For this review, use the dimensioned drawing (mm, ordinates from the lowest corner) and the shaded views. A direction names the side the tool comes from. Coordinates: 2 decimals unless noted, no trailing zeros. Loops run counter-clockwise (first coordinate to the right, second up) from the corner with the lowest first, then second, coordinate; pieces in that order, holes last. Notation, with made-up numbers: (-1, -37.75) - (16, -37.75) arc R23 cw to (16, -7.75) - close; hole circle Ø5 at (-0.5, -36). An arc over 180 degrees is marked (long way). Use one line per item in the form item = value. Start each with the question number.
(1) Clearance check with flat-ended pins moving along their axes: pin 1 Ø3 at (y, z) = (5.5, 25.5) entering from +X; pin 2 Ø0.9 at (x, z) = (16, 8.5) entering from +Y; pin 3 Ø3 at (x, z) = (16.5, 15) entering from -Y. State where each tip first meets the part, or that it passes through.
(2) Add section C-C (z = 23.75). State the section outline as (x, y) points.
(3) The part is to be moulded in two halves that separate along Z. For the marked faces 4, 5 and 6, say which applies: pulls with the +Z half, pulls with the -Z half, needs draft (parallel to the pull), parting line crosses it, or undercut.
(4) Add section D-D (y = 6.75). State the section outline as (x, z) points, plus the area to 3 significant figures.
(5) Tool access review of the marked faces 1, 2 and 3: name each direction out of +Z, -Z, +X, -X, +Y, -Y from which nothing blocks a thin tool from reaching the whole face with its end or side.
(6) Add section B-B (x = 16.5). State the section outline as (y, z) points, plus the area to 3 significant figures.
(7) For L1, parallel to Z at x = 16.5, y = 4.5; L2, parallel to Z at x = 16.5, y = 6.6; L3, parallel to X at y = 4, z = 15, list the stretches that pass through material, from the lowest coordinate up.
(8) Add section A-A (y = 4.5). State the section outline as (x, z) points.
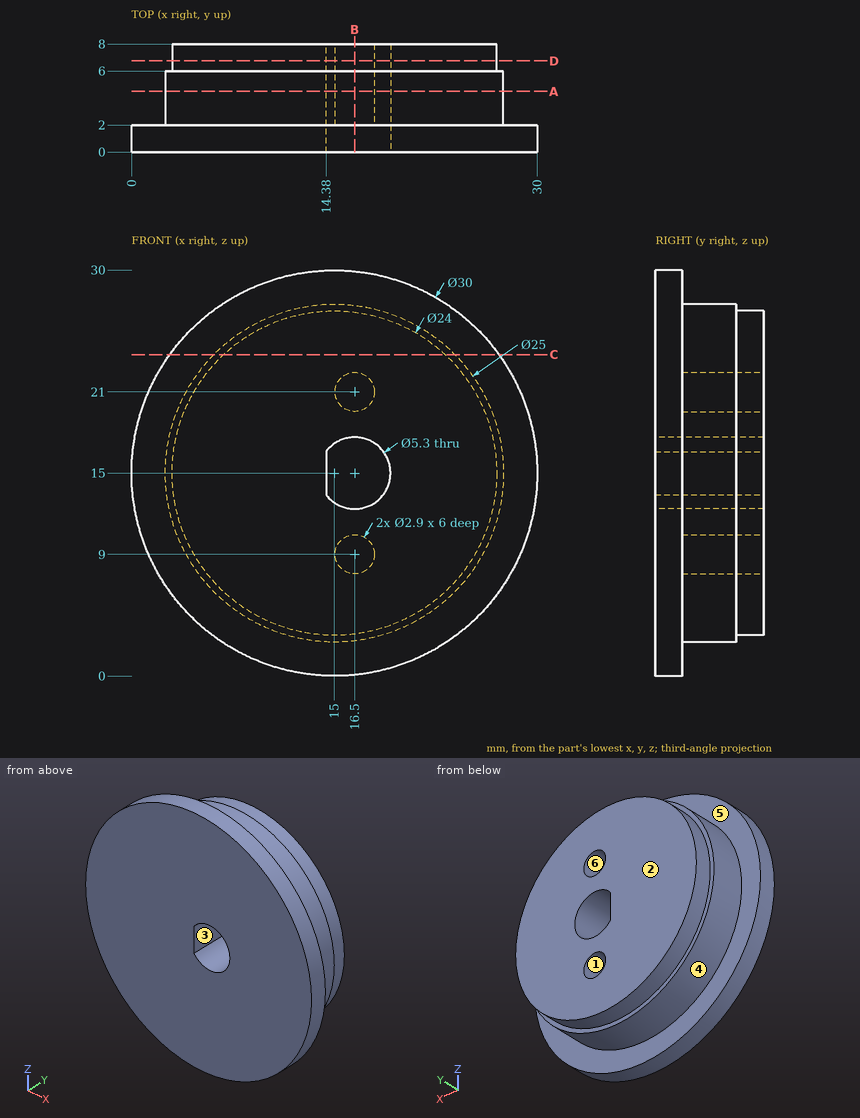
Computed values:
q1.pin_1 = 23.67
q1.pin_2 = 2
q1.pin_3 = through
q2.outline = (2.82, 0) - (27.18, 0) - (27.18, 2) - (23.93, 2) - (23.93, 6) - (23.21, 6) - (23.21, 8) - (6.79, 8) - (6.79, 6) - (6.07, 6) - (6.07, 2) - (2.82, 2) - close
q3.face_4 = parting line crosses it
q3.face_5 = needs draft
q3.face_6 = undercut
q4.outline = circle Ø24 at (15, 15); hole (14.38, 13.41) arc R2.65 ccw (long way) to (14.38, 16.59) - close; hole circle Ø2.9 at (16.5, 9); hole circle Ø2.9 at (16.5, 21)
q4.area = 418 mm^2
q5.face_1 = +Y
q5.face_2 = +Z, -Z, +X, -X, +Y
q5.face_3 = +Y, -Y
q6.outline = (0, 0.08) - (2, 0.08) - (2, 2.59) - (6, 2.59) - (6, 3.09) - (8, 3.09) - (8, 7.55) - (2, 7.55) - (2, 10.45) - (8, 10.45) - (8, 12.35) - (0, 12.35) - close; (0, 17.65) - (8, 17.65) - (8, 19.55) - (2, 19.55) - (2, 22.45) - (8, 22.45) - (8, 26.91) - (6, 26.91) - (6, 27.41) - (2, 27.41) - (2, 29.92) - (0, 29.92) - close
q6.area = 129 mm^2
q7.L1 = 2.59 to 7.55, 10.45 to 12.35, 17.65 to 19.55, 22.45 to 27.41
q7.L2 = 3.09 to 7.55, 10.45 to 12.35, 17.65 to 19.55, 22.45 to 26.91
q7.L3 = 2.5 to 14.38, 19.15 to 27.5
q8.outline = circle Ø25 at (15, 15); hole (14.38, 13.41) arc R2.65 ccw (long way) to (14.38, 16.59) - close; hole circle Ø2.9 at (16.5, 9); hole circle Ø2.9 at (16.5, 21)
